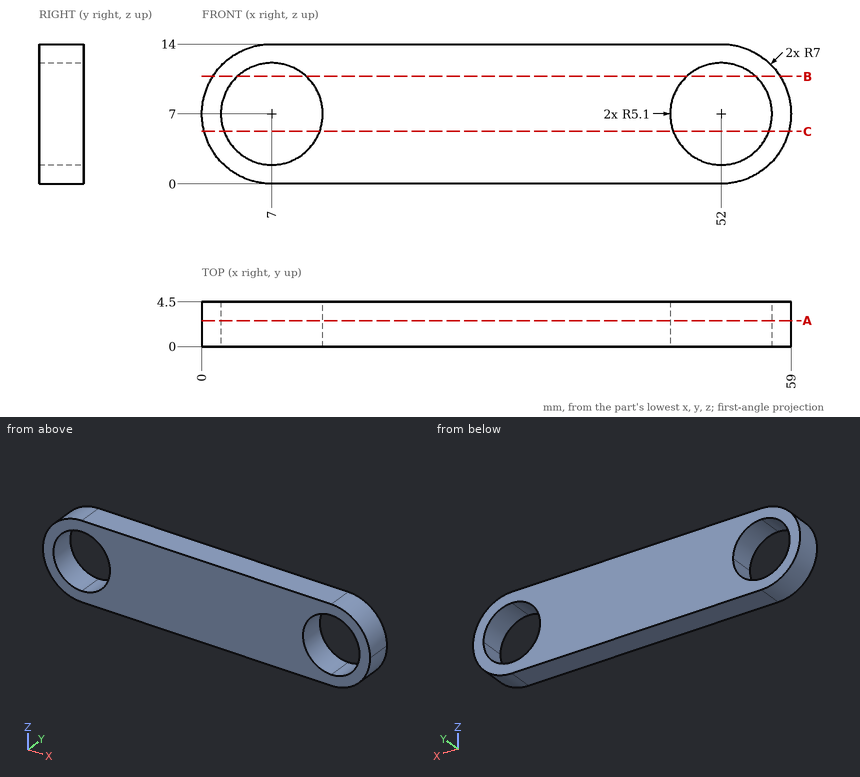
Print and shaded views of the part. All mm, measured from the part's lowest x, y and z. Coordinates: 2 decimals unless noted, no trailing zeros. Loops run counter-clockwise (first coordinate to the right, second up) from the corner with the lowest first, then second, coordinate; pieces in that order, holes last. Notation, with made-up numbers: M -17.75,62.5 L -4.75,62.5 A12 ccw -4.75,77.5 Z; hole C 23,43 d7. An arc over 180 degrees is marked long. Use a Markdown table: item, result. Add a question column.
Q1. Cut at C-C (z = 5.25). Write the cut outline in (x, y), and give its area (3 significant figures).
Q2. Cut at A-A (y = 2.6). Write the cut outline in (x, z).
Q3. Probe L1, parallel to X at y = 3.5, z = 7; L2, parallel to X at y = 0.85, z = 5.75; L3, parallel to Z at x = 49.5, y = 3.35. List the from-to ranges inside material, lowest first.
Q4. Cut at B-B (z = 10.75). Write the cut outline in (x, y), and give its area (3 significant figures).
Worked out:
| question | item | result |
|---|---|---|
| 1 | outline | M 0.22,0 L 2.21,0 L 2.21,4.5 L 0.22,4.5 Z; M 11.79,0 L 47.21,0 L 47.21,4.5 L 11.79,4.5 Z; M 56.79,0 L 58.78,0 L 58.78,4.5 L 56.79,4.5 Z |
| 1 | area | 177 mm2 |
| 2 | outline | M 7,0 L 52,0 A7 ccw 52,14 L 7,14 A7 ccw Z; hole C 7,7 d10.2; hole C 52,7 d10.2 |
| 3 | L1 | x = 0 to 1.9, 12.1 to 46.9, 57.1 to 59 |
| 3 | L2 | x = 0.11 to 2.06, 11.94 to 47.06, 56.94 to 58.89 |
| 3 | L3 | z = 0 to 2.55, 11.45 to 14 |
| 4 | outline | M 1.09,0 L 3.54,0 L 3.54,4.5 L 1.09,4.5 Z; M 10.46,0 L 48.54,0 L 48.54,4.5 L 10.46,4.5 Z; M 55.46,0 L 57.91,0 L 57.91,4.5 L 55.46,4.5 Z |
| 4 | area | 193 mm2 |
